from build123d import *

# Parameters (mm, degrees)
SKETCH_1_W          = 355
SKETCH_1_H          = 70
EXTRUDE_1_DEPTH     = 2
EXTRUDE_2_DEPTH     = 2
SKETCH_3_R          = 2
CUT_EXTRUDE_1_DEPTH = 195.38294737
SKETCH_4_R          = 1.5
CUT_EXTRUDE_2_DEPTH = 195.38294737
CUT_EXTRUDE_3_DEPTH = 2
CUT_EXTRUDE_4_DEPTH = 2
FILLET_1_R          = 10


with BuildPart() as part:
    # 草图1 → 凸台-拉伸1 (new body)
    with BuildSketch(Plane.XY):
        Rectangle(SKETCH_1_W, SKETCH_1_H)
    extrude(amount=EXTRUDE_1_DEPTH)

    # 草图2 → 凸台-拉伸2 (add)
    with BuildSketch(Plane.XY.offset(2)):
        Polygon((-12.5, -35), (-177.5, -79.211616751), (-177.5, -35), align=None)
    extrude(amount=-EXTRUDE_2_DEPTH)

    # 草图3 → 切除-拉伸1 (cut, through all)
    with BuildSketch(Plane.XY.offset(2)):
        with Locations((152.5, -30.5)):
            Circle(SKETCH_3_R)
        with Locations((24.5, -30.5)):
            Circle(SKETCH_3_R)
        with Locations((-103.5, -30.5)):
            Circle(SKETCH_3_R)
    extrude(amount=-CUT_EXTRUDE_1_DEPTH, mode=Mode.SUBTRACT)

    # 草图4 → 切除-拉伸2 (cut, through all)
    with BuildSketch(Plane.XY.offset(2)):
        with Locations((-97.127512474, -54.570045084)):
            Circle(SKETCH_4_R)
        with Locations((-88.434180038, -52.240673678)):
            Circle(SKETCH_4_R)
        with Locations((129.203708686, -10.489196039)):
            Circle(SKETCH_4_R)
        with Locations((158.181483474, -2.724624685)):
            Circle(SKETCH_4_R)
    extrude(amount=-CUT_EXTRUDE_2_DEPTH, mode=Mode.SUBTRACT)

    # 草图5 → 切除-拉伸3 (cut)
    with BuildSketch(Plane.XY.offset(2)):
        Polygon((-177.5, -5), (-28.217967697, 35), (-177.5, 35), align=None)
    extrude(amount=-CUT_EXTRUDE_3_DEPTH, mode=Mode.SUBTRACT)

    # 草图6 → 切除-拉伸4 (cut)
    with BuildSketch(Plane.XY.offset(2)):
        Polygon((-110.323085464, -61.211616751), (-177.5, -61.211616751), (-177.5, -79.211616751), align=None)
    extrude(amount=-CUT_EXTRUDE_4_DEPTH, mode=Mode.SUBTRACT)

    # 圆角1
    fillet_1_edges = [part.edges().sort_by_distance(p)[0] for p in [
        (-177.5, -5, 1),
        (-28.217967697, 35, 1),
        (-177.5, -61.211616751, 1),
        (177.5, -35, 1),
        (177.5, 35, 1),
    ]]
    fillet(fillet_1_edges, radius=FILLET_1_R)


solid = part.part
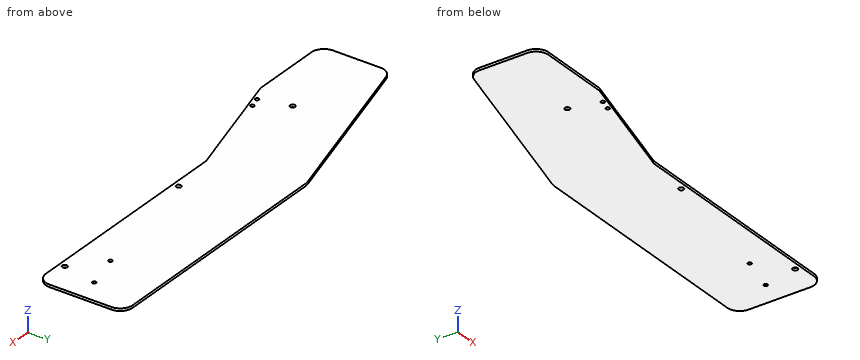
CAD build for the part. Positions are in the model's coordinates, mm. Round coordinates to 2 decimals unless told otherwise and drop trailing zeros. Write each loop counter-clockwise with the first axis right and the second up, starting at its lowest first coordinate (ties: lowest second). Pieces come first, ordered by that corner, then holes. Notation, with made-up numbers: M 61.25,22 L 107.25,22 A28 cw 107.25,46 Z; hole C 65,28.5 d5. An arc over 180 degrees is marked long. Put each result on its own line as item: value. Start each with the question number.
1) Saw through at C-C, the plane y = 29. Write the cut outline in (x, z), and give its area (3 significant figures).
2) Saw through at B-B, the plane x = 29.5. Write the cut outline in (y, z).
3) Saw through at A-A, the plane z = 0.35. Write the cut outline in (x, y), and give its area (3 significant figures).
4) Pin check, flat tips, straight feed: pin 1 Ø1.8 at (x, y) = (129.2, -10.49) entering from -Z; pin 2 Ø1 at (x, z) = (85, 1) entering from -Y. Stop position of each tip, or through.
5) Drill centre lines: probe 1 along X at (y, z) = (-31, 0.35); probe 2 along Y at (x, z) = (146, 0.35); probe 3 along Y at (x, z) = (-102, 0.65). Where is each one in solid material? Low to high. Write a range as [from, to].
Resolved:
1. outline: M -50.61,0 L 176.67,0 L 176.67,2 L -50.61,2 Z
1. area: 455 mm²
2. outline: M -35,0 L 35,0 L 35,2 L -35,2 Z
3. outline: M -177.5,-51.21 A10 ccw -167.5,-61.21 L -110.32,-61.21 L -12.5,-35 L 167.5,-35 A10 ccw 177.5,-25 L 177.5,25 A10 ccw 167.5,35 L -26.9,35 A10 ccw -29.49,34.66 L -170.09,-3.01 A10 ccw -177.5,-12.67 Z; hole C -103.5,-30.5 d4; hole C -97.13,-54.57 d3; hole C -88.43,-52.24 d3; hole C 24.5,-30.5 d4; hole C 129.2,-10.49 d3; hole C 152.5,-30.5 d4; hole C 158.18,-2.72 d3
3. area: 24,800 mm²
4. pin 1: through
4. pin 2: y = -35
5. probe 1: [-177.5, -105.44], [-101.56, 22.56], [26.44, 150.56], [154.44, 175.5]
5. probe 2: [-35, 35]
5. probe 3: [-58.98, -31.82], [-29.18, 15.23]
